Geometry check sheet. Reference: the model listing, model coordinates, mm. A direction names the side the tool comes from. Give positions to 0.01 mm unless a question says otherwise; leave off trailing zeros. Loops run counter-clockwise (first coordinate to the right, second up) from the corner with the lowest first, then second, coordinate; pieces in that order, holes last. Notation, with made-up numbers: (62.5, -2.5) -> (86.5, -2.5) arc R18 cw to (86.5, 24.5) -> close; hole circle Ø5 at (35, 17.5). An arc over 180 degrees is marked (long way). One line per item, written item: value. Start each with the question number.
(1) Draft check along X on faces 1 (the face through (-2, 239, 150)), 2 (the face through (-50, -15, 74)), 3 (the face through (-150, 231, -2)). Enter one of: pulls with the +X half, pulls with the -X half, needs draft (parallel to the pull), parting line crosses it, or undercut.
(2) Gauge pin test, flat ends, axial feed: pin 1 Ø8 at (x, z) = (12, 53) entering from -Y; pin 2 Ø9 at (x, y) = (-89, -10.5) entering from -Z; pin 3 Ø9 at (x, y) = (-9, -22.5) entering from +Z. Record the tip position at first contact, or that the pin passes through.
(3) Sectioned sample at B-B, the plane x = -14. Record the cut outline in (y, z), then the cut area to 4 significant figures.
(4) Tool access check on faces 4 (the face through (-1, 0, 74)), 5 (the face through (-101, 0, -76)), 6 (the face through (50, -15, -76)), 7 (the face through (150, 231, -2)). Record the directions out of +Z, -Z, +X, -X, +Y, -Y that give a thin tool (end or side, any length) a straight path to the whole face; none if there is none.
(5) Scan line: line 1 along Y through (x, z) = (-11, 133). Record every from-to range of solid material in increasing order. Write a range as from..to.
(6) Sectioned sample at C-C, the plane z = -118. Record the cut outline in (x, y), then the cut area to 3 significant figures.
(7) Sectioned sample at A-A, the plane z = 90. Record the cut outline in (x, y).
from build123d import *

# Parameters (mm, degrees)
BOX001_W     = 100
BOX001_H     = 30
BOX001_DEPTH = 150
BOX_W        = 300
BOX_H        = 500
BOX_DEPTH    = 300


with BuildPart() as cube001:
    # Box001 → Box001 (new body)
    with BuildSketch(Plane(origin=(50, -30, 0), x_dir=(1, 0, 0), z_dir=(0, 0, 1))):
        with Locations((50, 15)):
            Rectangle(BOX001_W, BOX001_H)
    extrude(amount=BOX001_DEPTH)


with BuildPart() as cube002:
    # Clone base: copy of Cube001
    add(cube001.part)


with BuildPart() as cube002_1:
    # Clone placement: moved
    add(cube002.part.moved(Location((-200, 0, 0))))


with BuildPart() as cube003:
    # Clone001 base: copy of Cube002
    add(cube002_1.part)


with BuildPart() as cube003_1:
    # Clone001 placement: moved
    add(cube003.part.moved(Location((100, 0, -150))))


with BuildPart() as fusion:
    # Box → Box (new body)
    with BuildSketch(Plane(origin=(-150, 0, -150), x_dir=(1, 0, 0), z_dir=(0, 0, 1))):
        with Locations((150, 250)):
            Rectangle(BOX_W, BOX_H)
    extrude(amount=BOX_DEPTH)

    # Fusion: union Cube001, Cube002, Cube003
    add(cube001.part)
    add(cube002_1.part)
    add(cube003_1.part)


solid = fusion.part
Calculated:
1. face 1: needs draft
1. face 2: undercut
1. face 3: pulls with the -X half
2. pin 1: stops at y = 0
2. pin 2: stops at z = 0
2. pin 3: stops at z = 0
3. outline: (-30, -150) -> (500, -150) -> (500, 150) -> (0, 150) -> (0, 0) -> (-30, 0) -> close
3. area: 154,500 mm2
4. face 4: +Z, -Y
4. face 5: -Z, -X, -Y
4. face 6: -Z, +X, -Y
4. face 7: +Z, -Z, +X, +Y, -Y
5. line 1: y = 0..500
6. outline: (-150, 0) -> (-50, 0) -> (-50, -30) -> (50, -30) -> (50, 0) -> (150, 0) -> (150, 500) -> (-150, 500) -> close
6. area: 153,000 mm2
7. outline: (-150, -30) -> (-50, -30) -> (-50, 0) -> (50, 0) -> (50, -30) -> (150, -30) -> (150, 500) -> (-150, 500) -> close
